The drawing under review shows one solid part. Ordinate dimensions are in mm from its lowest x, y, z. A direction names the side the tool comes from. Coordinates: 2 decimals unless noted, no trailing zeros. Loops run counter-clockwise (first coordinate to the right, second up) from the corner with the lowest first, then second, coordinate; pieces in that order, holes last. Notation, with made-up numbers: M -39.5,62.5 L -31.5,62.5 A26 ccw -31.5,81.5 Z; hole C 0,32.5 d1. An arc over 180 degrees is marked long. Put each result on its own line as item: value.
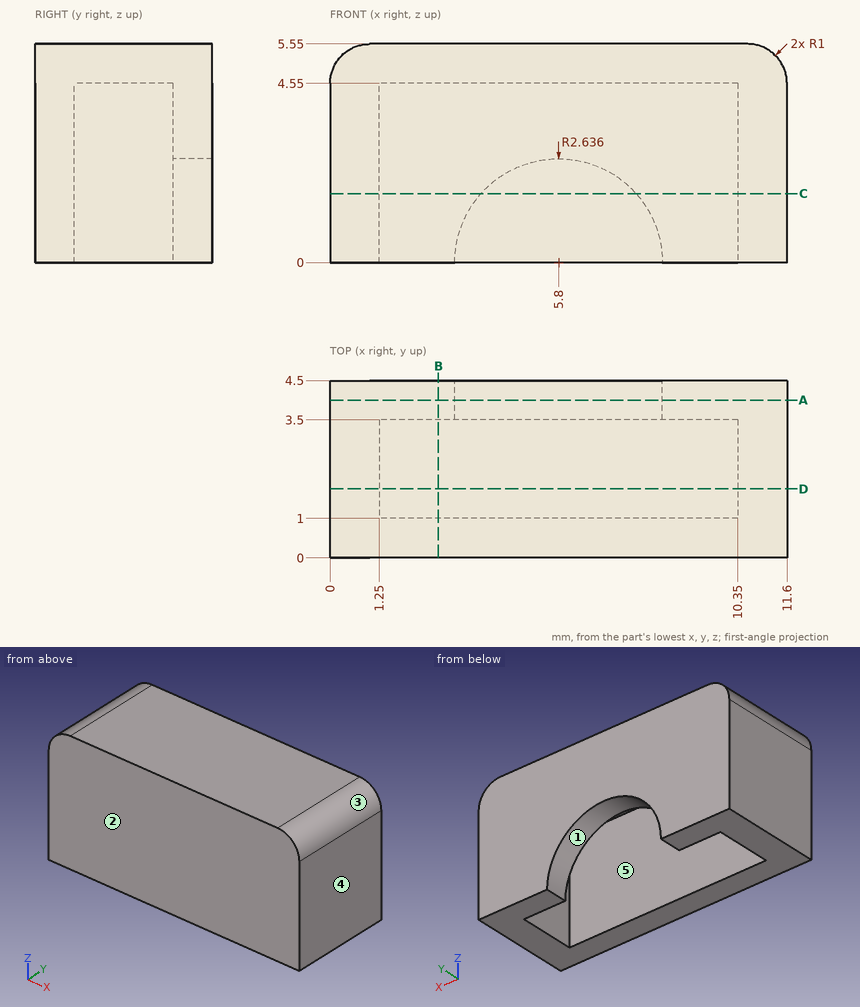
(1) For pin 1 (0.8 mm diameter, centred on x = 5, y = 2, fed in from -Z), flat-tipped, find the tip position at first contact; note if it passes through.
Determined:
pin 1: stops at z = 4.55
(2) Tool access review of the marked faces 4 and 5: name each direction out of +Z, -Z, +X, -X, +Y, -Y from which nothing blocks a thin tool from reaching the whole face with its end or side.
Determined:
face 4: +Z, -Z, +X, +Y, -Y
face 5: -Z
(3) Wall thickness on line 1 along X through (y, z) = (2.45, 4.05); line 2 along Y through (x, z) = (10, 3.6); line 3 along Z through (x, y) = (8.5, 1.2): over which ranges is each line inside the solid? List them lowest first. Write a range as [from, to].
Determined:
line 1: x = [0, 1.25], [10.35, 11.6]
line 2: y = [0, 1], [3.5, 4.5]
line 3: z = [4.55, 5.55]
(4) Add section D-D (y = 1.75). Write out the cut boundary in (x, z).
Determined:
outline: M 0,0 L 1.25,0 L 1.25,4.55 L 10.35,4.55 L 10.35,0 L 11.6,0 L 11.6,4.55 A1 ccw 10.6,5.55 L 1,5.55 A1 ccw 0,4.55 Z
(5) Add section B-B (x = 2.75). Write out the cut boundary in (y, z), plus the area to 3 significant figures.
Determined:
outline: M 0,0 L 1,0 L 1,4.55 L 3.5,4.55 L 3.5,0 L 4.5,0 L 4.5,5.55 L 0,5.55 Z
area: 13.6 mm^2
(6) Add section C-C (z = 1.75). Write out the cut boundary in (x, y), plus the area to 3 significant figures.
Determined:
outline: M 0,0 L 11.6,0 L 11.6,4.5 L 7.77,4.5 L 7.77,3.5 L 10.35,3.5 L 10.35,1 L 1.25,1 L 1.25,3.5 L 3.83,3.5 L 3.83,4.5 L 0,4.5 Z
area: 25.5 mm^2
(7) Add section A-A (y = 4). Write out the cut boundary in (x, z).
Determined:
outline: M 0,0 L 3.16,0 A2.64 cw 8.44,0 L 11.6,0 L 11.6,4.55 A1 ccw 10.6,5.55 L 1,5.55 A1 ccw 0,4.55 Z
(8) Draft analysis for pull direction X (two halves, no side actions). For the marked faces 1, 2 and 3, state which applies: +X half, -X half, draft (parallel to the pull), parting line (faces both ways), or undercut.
Determined:
face 1: undercut
face 2: draft
face 3: +X half
